Design review of the part built by this model. Coordinates are the model's own, in mm. A direction names the side the tool comes from. Give positions to 0.01 mm unless a question says otherwise; leave off trailing zeros. Loops run counter-clockwise (first coordinate to the right, second up) from the corner with the lowest first, then second, coordinate; pieces in that order, holes last. Notation, with made-up numbers: (81, -40) - (109, -40) arc R24 ccw to (109, -14) - close; hole circle Ø1 at (-8, 64). An arc over 180 degrees is marked (long way). Write each question's results on one line, items separated by ' | '.
```python
from build123d import *

# Parameters (mm, degrees)
F0_R     = 15
F1_DEPTH = 10
F1_TAPER = 12
F2_R     = 8
F3_DEPTH = 6
F3_TAPER = 3
F4_R     = 1.725
F5_DEPTH = 4


with BuildPart() as f1:
    # F0 (on Top) → F1 (new body)
    with BuildSketch(Plane.XY):
        Circle(F0_R)
    extrude(amount=F1_DEPTH, taper=F1_TAPER)

    # F2 (on face) → F3 (cut)
    with BuildSketch(Plane.XY.offset(10)):
        Circle(F2_R)
    extrude(amount=-F3_DEPTH, taper=F3_TAPER, mode=Mode.SUBTRACT)

    # F4 (on face) → F5 (cut, through all)
    with BuildSketch(Plane.XY.offset(4)):
        Circle(F4_R)
    extrude(amount=-F5_DEPTH, mode=Mode.SUBTRACT)


solid = f1.part
```
Item 1: We need section A-A on x = 0. Give the boundary of the cut face in (y, z) (3 decimals), then the cut area to 3 significant figures.
Output values:
outline: (-15, 0) - (-1.725, 0) - (-1.725, 4) - (-7.686, 4) - (-8, 10) - (-12.874, 10) - close; (1.725, 0) - (15, 0) - (12.874, 10) - (8, 10) - (7.686, 4) - (1.725, 4) - close | area: 171 mm²
Item 2: Clearance check with flat-ended pins moving along their axes: P1, Ø4.5, axis at x = 0, y = 0, coming from the +Z side; P2, Ø4, axis at x = -9.5, z = 3.5, coming from the -Y side; P3, Ø3, axis at y = 7, z = 4, coming from the +X side. State where each tip first meets the part, or that it passes through.
Output values:
P1: stops at z = 4 | P2: stops at y = -12.22 | P3: stops at x = 13.12
Item 3: Draft analysis for pull direction X (two halves, no side actions). For faces 1 (the face through (-2.86, -12.9, 8.4)), 2 (the face through (-0.22, 1.71, 2.03)), 3 (the face through (0, -3, 0)), state which applies: +X half, -X half, draft (parallel to the pull), parting line (faces both ways), or undercut.
Output values:
face 1: parting line | face 2: undercut | face 3: draft
Item 4: Tool access review of faces 4 (the face through (0, 2, 4)), 5 (the face through (-6, -6, 10)): name each direction out of +Z, -Z, +X, -X, +Y, -Y from which nothing blocks a thin tool from reaching the whole face with its end or side.
Output values:
face 4: +Z | face 5: +Z, +X, -X, +Y, -Y
Item 5: Wall thickness on probe 1 along Y at (x, z) = (-3, 7); probe 2 along Y at (x, z) = (2.5, 9); probe 3 along Z at (x, y) = (1, -2): over which ranges is each line inside the solid? List them lowest first.
Output values:
probe 1: y = -13.17 to -7.25, 7.25 to 13.17 | probe 2: y = -12.85 to -7.54, 7.54 to 12.85 | probe 3: z = 0 to 4
